Verification items for the finished model (mm, model axes). A direction names the side the tool comes from. Round coordinates to 2 decimals unless told otherwise and drop trailing zeros. One line per item, written item: value. Start each with the question number.
Item 1: Gauge pin test, flat ends, axial feed: pin 1 (4 mm diameter, centred on y = 115.5, z = -42.5, fed in from +X); pin 2 (6 mm diameter, centred on y = 86.5, z = -68.5, fed in from -X); pin 3 (10 mm diameter, centred on x = -12.5, y = -7, fed in from -Z). Record the tip position at first contact, or that the pin passes through.
Item 2: Section check A-A, the plane x = 1. State how many separate pieces and enclosed holes the cut face has, then the cut area to 3 significant figures.
Item 3: Draft check along Z on faces 4 (the face through (-19.48, 41.655, 0.71)), 5 (the face through (17.446, 8.56, -12.254)), 6 (the face through (-21.5, -26.38, 28.63)). Enter one of: +Z half, -Z half, draft (parallel to the pull), parting line (faces both ways), or undercut.
Item 4: Tool access check on faces 1 (the face through (24.78, 59.49, 48.64)), 2 (the face through (-5.88, 58.89, -105.13)), 3 (the face through (54.87, -14.16, -20.74)). Record the directions out of +Z, -Z, +X, -X, +Y, -Y that give a thin tool (end or side, any length) a straight path to the whole face; none if there is none.
Item 5: Thickness scan on probe 1 along Z at (x, y) = (14, 72.5); probe 2 along Y at (x, z) = (16.5, -29.5); probe 3 along Z at (x, y) = (7, 110). Record the ranges inside material, lowest first. Write a range as from..to.
from build123d import *


with BuildPart() as f1:
    # F0 (on Top) → F1 (revolve)
    with BuildSketch(Plane.XY):
        Polygon((-46.406250447, 20.1154891402), (-30.5095128715, -21.2160330266), (-34.9116884172, -22.9279901832), (-43.2269051671, -19.9932083488), (-53.7432096899, -12.9008162767), (-64.0149489045, -7.0312502794), (-66.7051672935, -18.7703818083), (-66.7051672935, -38.0910336971), (-41.2703827024, -38.0910336971), (-19.7850654535, -31.732339412), (-21.4605983347, -28.308423236), (-9.9660325795, -22.6834248751), (8.3763608709, -16.5907324904), (-10.6997303665, -33.6888581514), (-5.5638612248, -60.1207125871), (15.9578826278, -60.1207125871), (42.7095489145, -60.1207125871), (66.5828809142, -44.2051626742), (58.2676678896, -31.732339412), (55.0883151591, -16.5907324904), (49.2665074484, -7.5181558132), (46.7730984092, -7.2758155875), (44.4394518833, -31.2864202052), (39.1915775836, -42.2486439347), (16.2024479359, -31.2432069331), (33.0919572228, -16.5907324904), (37.4796167016, -14.8573378101), (31.6100567579, 0), (16.9552299565, 7.0306546103), (14.9796204641, 11.3111417741), (34.0557061136, 20.1154891402), (34.0557061136, 36.0122285783), (11.3111417741, 47.0176674426), (-15.5910328031, 43.8383184373), (-25.3736432642, 37.9687510431), (-22.2819369673, 30.0316486084), (-21.4605983347, 23.0502728373), align=None)
    revolve(axis=Axis((-2.1399455145, 45.4279929399, 0), (0.9930888363, 0.1173650849, 0)))


solid = f1.part
Response values:
1. pin 1: stops at x = 40.42
1. pin 2: stops at x = -24.94
1. pin 3: stops at z = -93.81
2. separate pieces: 1
2. enclosed holes: 2
2. area: 35,100 mm2
3. face 4: undercut
3. face 5: undercut
3. face 6: parting line
4. face 1: none
4. face 2: -X
4. face 3: +X
5. probe 1: z = -105.64..-80.84, -67..-35.46, -22.86..22.86, 35.46..67, 80.84..105.64
5. probe 2: y = -56..-26.02, -24.6..18.99, 29.2..63.42, 82.81..108.17, 134.06..154.32
5. probe 3: z = -87.99..-53.98, -37.26..37.26, 53.98..87.99
